```python
from build123d import *

# Parameters (mm, degrees)
SKETCH_2_W           = 80
SKETCH_2_H           = 34
SKETCH_2_R           = 4.05
EXTRUDE_1_DEPTH      = 8
SKETCH_3_R           = 2.55
CUT_EXTRUDE_1_DEPTH  = 88.292611371
CUT_EXTRUDE_2_DEPTH  = 88.292611371
SKETCH_5_R           = 1.55
CUT_EXTRUDE_3_DEPTH  = 88.292611371
CUT_EXTRUDE_5_DEPTH  = 4.5
SKETCH_25_R          = 1.55
CUT_EXTRUDE_13_DEPTH = 88.292611371
CUT_EXTRUDE_11_DEPTH = 2
EXTRUDE_2_DEPTH      = 8
SKETCH_26_R          = 5.025
CUT_EXTRUDE_14_DEPTH = 89.926936302
SKETCH_27_R          = 2.9
SKETCH_27_R_2        = 1.55
CUT_EXTRUDE_15_DEPTH = 89.926936302
CUT_EXTRUDE_16_DEPTH = 6
SKETCH_29_R          = 5.5
CUT_EXTRUDE_17_DEPTH = 89.926936302


with BuildPart() as part:
    # Sketch 2 → Extrude 1 (new body)
    with BuildSketch(Plane.XY):
        with Locations((40, 17)):
            Rectangle(SKETCH_2_W, SKETCH_2_H)
        with Locations((7, 8)):
            Circle(SKETCH_2_R, mode=Mode.SUBTRACT)
        with Locations((40, 10)):
            Circle(SKETCH_2_R, mode=Mode.SUBTRACT)
        with Locations((73, 8)):
            Circle(SKETCH_2_R, mode=Mode.SUBTRACT)
    extrude_1 = extrude(amount=EXTRUDE_1_DEPTH)

    # Sketch 3 → Cut-Extrude 1 (cut, through all)
    with BuildSketch(Plane.XY.offset(8)):
        with Locations((23, 8)):
            Circle(SKETCH_3_R)
        with Locations((57, 8)):
            Circle(SKETCH_3_R)
    extrude(amount=-CUT_EXTRUDE_1_DEPTH, mode=Mode.SUBTRACT)

    # Sketch 4 → Cut-Extrude 2 (cut, through all)
    with BuildSketch(Plane(origin=(80, 0, 0), x_dir=(0, 0, -1), z_dir=(1, 0, 0))):
        Polygon((-1.5, 32.2), (-2.5, 32.2), (-2.5, 34), (0, 34), (0, 28.8), (-1.5, 28.8), align=None)
    cut_extrude_2 = extrude(amount=-CUT_EXTRUDE_2_DEPTH, mode=Mode.SUBTRACT)

    # Sketch 5 → Cut-Extrude 3 (cut, through all)
    with BuildSketch(Plane.XY.offset(8)):
        with Locations((48, 10)):
            Circle(SKETCH_5_R)
        with Locations((32, 10)):
            Circle(SKETCH_5_R)
    cut_extrude_3 = extrude(amount=-CUT_EXTRUDE_3_DEPTH, mode=Mode.SUBTRACT)

    # Sketch 8 → Cut-Extrude 5 (cut)
    with BuildSketch(Plane(origin=(0, 0, 0), x_dir=(-1, 0, 0), z_dir=(0, 0, -1))):
        Polygon((-45.15, 8.354551733), (-45.15, 11.645448267), (-48, 13.290896534), (-50.85, 11.645448267), (-50.85, 8.354551733), (-48, 6.709103466), align=None)
        Polygon((-29.15, 8.354551733), (-29.15, 11.645448267), (-32, 13.290896534), (-34.85, 11.645448267), (-34.85, 8.354551733), (-32, 6.709103466), align=None)
    cut_extrude_5 = extrude(amount=-CUT_EXTRUDE_5_DEPTH, mode=Mode.SUBTRACT)

    # Sketch 25 → Cut-Extrude 13 (cut, through all)
    with BuildSketch(Plane(origin=(0, 0, 0), x_dir=(-1, 0, 0), z_dir=(0, 0, -1))):
        with Locations((-60, 25)):
            Circle(SKETCH_25_R)
        with Locations((-20, 25)):
            Circle(SKETCH_25_R)
    cut_extrude_13 = extrude(amount=-CUT_EXTRUDE_13_DEPTH, mode=Mode.SUBTRACT)

    # Sketch 19 → Cut-Extrude 11 (cut)
    with BuildSketch(Plane(origin=(0, 0, 2.5), x_dir=(-1, 0, 0), z_dir=(0, 0, -1))):
        with BuildLine():
            Line((-25, 34), (-55.247938178, 34))
            Line((-55.247938178, 34), (-55.247938178, 33.2))
            ThreePointArc((-55.247938178, 33.2), (-54.747938178, 32.7), (-54.247938178, 33.2))
            Line((-54.247938178, 33.2), (-26, 33.2))
            ThreePointArc((-26, 33.2), (-25.5, 32.7), (-25, 33.2))
            Line((-25, 33.2), (-25, 34))
        make_face()
    cut_extrude_11 = extrude(amount=-CUT_EXTRUDE_11_DEPTH, mode=Mode.SUBTRACT)

    # Sketch 22 → Extrude 2 (add)
    with BuildSketch(Plane.XY.offset(8)):
        with BuildLine():
            Line((0, -4), (5.5, -4))
            ThreePointArc((5.5, -4), (3.5, -2), (5.5, 0))
            Line((5.5, 0), (0, 0))
            ThreePointArc((0, 0), (2, -2), (0, -4))
        make_face()
        with BuildLine():
            Line((80, 0), (74.5, 0))
            ThreePointArc((74.5, 0), (76.5, -2), (74.5, -4))
            Line((74.5, -4), (80, -4))
            ThreePointArc((80, -4), (78, -2), (80, 0))
        make_face()
    extrude(amount=-EXTRUDE_2_DEPTH)

    # Mirror 2: Extrude 1, Cut-Extrude 2, Cut-Extrude 3, Cut-Extrude 5, Cut-Extrude 13, Cut-Extrude 11 across plane
    add(extrude_1.mirror(Plane(origin=(0, -2, 0), x_dir=(0, 0, 1), z_dir=(0, -1, 0))))
    add(cut_extrude_2.mirror(Plane(origin=(0, -2, 0), x_dir=(0, 0, 1), z_dir=(0, -1, 0))), mode=Mode.SUBTRACT)
    add(cut_extrude_3.mirror(Plane(origin=(0, -2, 0), x_dir=(0, 0, 1), z_dir=(0, -1, 0))), mode=Mode.SUBTRACT)
    add(cut_extrude_5.mirror(Plane(origin=(0, -2, 0), x_dir=(0, 0, 1), z_dir=(0, -1, 0))), mode=Mode.SUBTRACT)
    add(cut_extrude_13.mirror(Plane(origin=(0, -2, 0), x_dir=(0, 0, 1), z_dir=(0, -1, 0))), mode=Mode.SUBTRACT)
    add(cut_extrude_11.mirror(Plane(origin=(0, -2, 0), x_dir=(0, 0, 1), z_dir=(0, -1, 0))), mode=Mode.SUBTRACT)

    # Sketch 26 → Cut-Extrude 14 (cut, through all)
    with BuildSketch(Plane(origin=(0, 0, 0), x_dir=(-1, 0, 0), z_dir=(0, 0, -1))):
        with Locations((-73, -12)):
            Circle(SKETCH_26_R)
        with Locations((-7, -12)):
            Circle(SKETCH_26_R)
    extrude(amount=-CUT_EXTRUDE_14_DEPTH, mode=Mode.SUBTRACT)

    # Sketch 27 → Cut-Extrude 15 (cut, through all)
    with BuildSketch(Plane(origin=(0, 0, 0), x_dir=(-1, 0, 0), z_dir=(0, 0, -1))):
        with Locations((-66.2, 11.5)):
            Circle(SKETCH_27_R)
        with Locations((-66.2, -15.5)):
            Circle(SKETCH_27_R_2)
        with Locations(Location((-13.8, -15.5, 0), (0, 0, 180))):
            Circle(SKETCH_27_R_2)
        with Locations(Location((-13.8, 11.5, 0), (0, 0, 180))):
            Circle(SKETCH_27_R)
    extrude(amount=-CUT_EXTRUDE_15_DEPTH, mode=Mode.SUBTRACT)

    # Sketch 28 → Cut-Extrude 16 (cut)
    with BuildSketch(Plane(origin=(0, 0, 0), x_dir=(-1, 0, 0), z_dir=(0, 0, -1))):
        Polygon((-52.9, 5.632863896), (-52.9, 10.367136104), (-57, 12.734272207), (-61.1, 10.367136104), (-61.1, 5.632863896), (-57, 3.265727793), align=None)
        Polygon((-18.9, 5.632863896), (-18.9, 10.367136104), (-23, 12.734272207), (-27.1, 10.367136104), (-27.1, 5.632863896), (-23, 3.265727793), align=None)
    extrude(amount=-CUT_EXTRUDE_16_DEPTH, mode=Mode.SUBTRACT)

    # Sketch 29 → Cut-Extrude 17 (cut, through all)
    with BuildSketch(Plane(origin=(0, 0, 0), x_dir=(-1, 0, 0), z_dir=(0, 0, -1))):
        with Locations((-40, -14)):
            Circle(SKETCH_29_R)
    extrude(amount=-CUT_EXTRUDE_17_DEPTH, mode=Mode.SUBTRACT)


solid = part.part
```
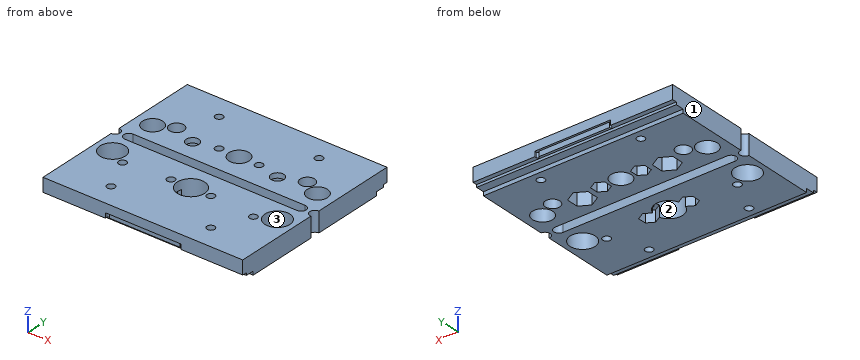
Can you work these out from the model? Positions are in its coordinate system, mm. Face numbers are marked on the shaded views. Round coordinates to 2 decimals unless told otherwise and drop trailing zeros. Loops run counter-clockwise (first coordinate to the right, second up) from the corner with the lowest first, then second, coordinate; pieces in that order, holes last. Notation, with made-up numbers: M 62,35 L 92,35 A35 cw 92,74 Z; hole C 12,18.25 d7. An arc over 180 degrees is marked long. Write item = value, one per line. Start each with the question number.
(1) If we mould it in two halves opening along Y, with no side actions, what happens to the marked faces 1, 2 and 3? For each: released by +Y, released by -Y, zero draft, split by the parting line, or undercut.
(2) I need wall thicknesses on line 1 along Y through (x, z) = (60, 6.25); line 2 along Y through (x, z) = (57, 6.6); line 3 along Y through (x, z) = (13.8, 2.75). Which ranges of each line are inside material? Lowest first, please.
(3) Suppose I cut it at A-A on x = 7. Write out the boundary of the cut face in (y, z) (3 decimals), plus the area to 3 significant figures.
(4) I'm going to push flat-ended pins straight in: P1, Ø3.5, axis at x = 32, y = 10, coming from the -Z side; P2, Ø2, axis at x = 45.5, y = -37, coming from the -Z side. Where does each tip first touch, or does it pass through?
(5) Suppose I cut it at B-B on x = 71. Write out the boundary of the cut face in (y, z), plus the area to 3 significant figures.
Answer block:
q1.face_1 = zero draft
q1.face_2 = undercut
q1.face_3 = undercut
q2.line_1 = -38 to -30.55, -27.45 to -4, 0 to 23.45, 26.55 to 34
q2.line_2 = -38 to -4, 0 to 5.45, 10.55 to 34
q2.line_3 = -38 to -17.05, -13.95 to -4, 0 to 8.6, 14.4 to 34
q3.outline = M -38,2.5 L -36.2,2.5 L -36.2,1.5 L -32.8,1.5 L -32.8,0 L -17.025,0 L -17.025,8 L -38,8 Z; M -6.975,0 L -4,0 L -4,8 L -6.975,8 Z; M 0,0 L 3.95,0 L 3.95,8 L 0,8 Z; M 12.05,0 L 28.8,0 L 28.8,1.5 L 32.2,1.5 L 32.2,2.5 L 34,2.5 L 34,8 L 12.05,8 Z
q3.area = 380 mm²
q4.P1 = 4.5
q4.P2 = 1.5
q5.outline = M -38,2.5 L -36.2,2.5 L -36.2,1.5 L -32.8,1.5 L -32.8,0 L -16.61,0 L -16.61,8 L -38,8 Z; M -7.39,0 L -4,0 L -4,8 L -7.39,8 Z; M 0,0 L 4.48,0 L 4.48,8 L 0,8 Z; M 11.52,0 L 28.8,0 L 28.8,1.5 L 32.2,1.5 L 32.2,2.5 L 34,2.5 L 34,8 L 11.52,8 Z
q5.area = 395 mm²
